from build123d import *

# Parameters (mm, degrees)
F0_W     = 195
F0_H     = 49
F0_R     = 1.25
F0_R_2   = 2.4
F0_R_3   = 3.1
F0_R_4   = 3.5
F0_R_5   = 1
F0_R_6   = 2.25
F0_R_7   = 2.6
F0_R_8   = 3
F1_DEPTH = 25
F2_DEPTH = 10
F3_DEPTH = 15
F4_DEPTH = 7


with BuildPart() as f1:
    # F0 (on Top) → F1 (new body)
    with BuildSketch(Plane.XY):
        with Locations((97.5, 24.5)):
            Rectangle(F0_W, F0_H)
        with Locations((27.5, 16.333333)):
            Circle(F0_R, mode=Mode.SUBTRACT)
        with Locations((47.5, 16.333333)):
            Circle(F0_R, mode=Mode.SUBTRACT)
        with Locations((67.5, 16.333333)):
            Circle(F0_R_2, mode=Mode.SUBTRACT)
        with Locations((87.5, 16.333333)):
            Circle(F0_R_2, mode=Mode.SUBTRACT)
        with Locations((107.5, 16.333333)):
            Circle(F0_R_3, mode=Mode.SUBTRACT)
        with Locations((127.5, 16.333333)):
            Circle(F0_R_3, mode=Mode.SUBTRACT)
        with Locations((147.5, 16.333333)):
            Circle(F0_R_4, mode=Mode.SUBTRACT)
        with Locations((167.5, 16.333333)):
            Circle(F0_R_4, mode=Mode.SUBTRACT)
        with Locations((27.5, 32.666667)):
            Circle(F0_R_5, mode=Mode.SUBTRACT)
        with Locations((47.5, 32.666667)):
            Circle(F0_R_5, mode=Mode.SUBTRACT)
        with Locations((67.5, 32.666667)):
            Circle(F0_R_6, mode=Mode.SUBTRACT)
        with Locations((87.5, 32.666667)):
            Circle(F0_R_6, mode=Mode.SUBTRACT)
        with Locations((107.5, 32.666667)):
            Circle(F0_R_7, mode=Mode.SUBTRACT)
        with Locations((127.5, 32.666667)):
            Circle(F0_R_7, mode=Mode.SUBTRACT)
        with Locations((147.5, 32.666667)):
            Circle(F0_R_8, mode=Mode.SUBTRACT)
        with Locations((167.5, 32.666667)):
            Circle(F0_R_8, mode=Mode.SUBTRACT)
        with Locations((27.5, 32.666667)):
            Circle(F0_R_5)
        with Locations((27.5, 16.333333)):
            Circle(F0_R)
        with Locations((47.5, 16.333333)):
            Circle(F0_R)
        with Locations((47.5, 32.666667)):
            Circle(F0_R_5)
        with Locations((67.5, 32.666667)):
            Circle(F0_R_6)
        with Locations((67.5, 16.333333)):
            Circle(F0_R_2)
        with Locations((87.5, 32.666667)):
            Circle(F0_R_6)
        with Locations((87.5, 16.333333)):
            Circle(F0_R_2)
        with Locations((107.5, 16.333333)):
            Circle(F0_R_3)
        with Locations((107.5, 32.666667)):
            Circle(F0_R_7)
        with Locations((147.5, 32.666667)):
            Circle(F0_R_8)
        with Locations((127.5, 32.666667)):
            Circle(F0_R_7)
        with Locations((127.5, 16.333333)):
            Circle(F0_R_3)
        with Locations((147.5, 16.333333)):
            Circle(F0_R_4)
        with Locations((167.5, 32.666667)):
            Circle(F0_R_8)
        with Locations((167.5, 16.333333)):
            Circle(F0_R_4)
    extrude(amount=-F1_DEPTH)

    # F0 (on Top) → F2 (cut)
    with BuildSketch(Plane.XY):
        with Locations((27.5, 32.666667)):
            Circle(F0_R_5)
        with Locations((47.5, 32.666667)):
            Circle(F0_R_5)
        with Locations((27.5, 16.333333)):
            Circle(F0_R)
        with Locations((47.5, 16.333333)):
            Circle(F0_R)
        with Locations((107.5, 32.666667)):
            Circle(F0_R_7)
        with Locations((107.5, 16.333333)):
            Circle(F0_R_3)
        with Locations((127.5, 32.666667)):
            Circle(F0_R_7)
        with Locations((127.5, 16.333333)):
            Circle(F0_R_3)
    extrude(amount=-F2_DEPTH, mode=Mode.SUBTRACT)

    # F0 (on Top) → F3 (cut)
    with BuildSketch(Plane.XY):
        with Locations((67.5, 32.666667)):
            Circle(F0_R_6)
        with Locations((87.5, 32.666667)):
            Circle(F0_R_6)
        with Locations((87.5, 16.333333)):
            Circle(F0_R_2)
        with Locations((67.5, 16.333333)):
            Circle(F0_R_2)
    extrude(amount=-F3_DEPTH, mode=Mode.SUBTRACT)

    # F0 (on Top) → F4 (cut)
    with BuildSketch(Plane.XY):
        with Locations((147.5, 32.666667)):
            Circle(F0_R_8)
        with Locations((147.5, 16.333333)):
            Circle(F0_R_4)
        with Locations((167.5, 16.333333)):
            Circle(F0_R_4)
        with Locations((167.5, 32.666667)):
            Circle(F0_R_8)
    extrude(amount=-F4_DEPTH, mode=Mode.SUBTRACT)


solid = f1.part
Verification items for the finished model (mm, model axes). A direction names the side the tool comes from. Coordinates: 2 decimals unless noted, no trailing zeros. Order: outer loops, then holes, each group sorted by start corner. A loop starts at its lowest first (then second) coordinate and runs counter-clockwise, first axis right, second up.
1. Set-up check for faces 4 (the face through (96, 25, 0)), 5 (the face through (87, 16, -15)): record each of +Z, -Z, +X, -X, +Y, -Y from which the full face is reachable in a straight line by a thin tool's end or side.
Results found:
face 4: +Z, +X, -X, +Y, -Y
face 5: +Z
2. Scan lines: line 1 (Y direction, x = 87.5, z = -3.75); line 2 (Y direction, x = 127.5, z = -4.25); line 3 (X direction, y = 32, z = -11). Record each from-to range of solid material in increasing order.
Results found:
line 1: y = 0 to 13.93, 18.73 to 30.42, 34.92 to 49
line 2: y = 0 to 13.23, 19.43 to 30.07, 35.27 to 49
line 3: x = 0 to 65.35, 69.65 to 85.35, 89.65 to 195
3. Release check for a two-part mould opening along X. For faces 1 (the face through (96, 49, -12)), 2 (the face through (147, 16, -7)), 3 (the face through (127, 33, -10)) record: +X half, -X half, draft (parallel to the pull), parting line (faces both ways), or undercut.
Results found:
face 1: draft
face 2: undercut
face 3: undercut
4. Sectioned sample at B-B, the plane x = 107.5. Record the cut outline in (y, z), and give its area (3 significant figures).
Results found:
outline: (0, -25) - (49, -25) - (49, 0) - (35.27, 0) - (35.27, -10) - (30.07, -10) - (30.07, 0) - (19.43, 0) - (19.43, -10) - (13.23, -10) - (13.23, 0) - (0, 0) - close
area: 1,110 mm2
5. Go/stop test with flat-tipped pins: pin 1 Ø1.9 at (x, y) = (107, 17.5) entering from +Z; pin 2 Ø2 at (x, y) = (168.5, 14.5) entering from +Z; pin 3 Ø3 at (x, y) = (67.5, 16.33) entering from +Z. Record where each tip stops, or that it passes through.
Results found:
pin 1: stops at z = -10
pin 2: stops at z = -7
pin 3: stops at z = -15
6. Sectioned sample at A-A, the plane x = 147.5. Record the cut outline in (y, z), and give its area (3 significant figures).
Results found:
outline: (0, -25) - (49, -25) - (49, 0) - (35.67, 0) - (35.67, -7) - (29.67, -7) - (29.67, 0) - (19.83, 0) - (19.83, -7) - (12.83, -7) - (12.83, 0) - (0, 0) - close
area: 1,130 mm2
